Design review of the part shown in the three views and the two pictorial views. Dimensions are in mm from the part's minimum x, y and z. Give positions to 0.01 mm unless a question says otherwise; leave off trailing zeros. Loops run counter-clockwise (first coordinate to the right, second up) from the corner with the lowest first, then second, coordinate; pieces in that order, holes last. Notation, with made-up numbers: (-30, 42) -> (-4, 42) arc R5 ccw to (-4, 48) -> close; hole circle Ø8 at (21.5, 42). An arc over 180 degrees is marked (long way). One line per question, with ' | ' between items. Start each with the question number.
(1) Consider section A-A (z = 30.5). Write out the cut boundary in (x, y), and give its area (3 significant figures).
(2) Wall thickness on probe 1 along Y at (x, z) = (10, 77); probe 2 along X at (y, z) = (8.5, 61.5); probe 3 along Z at (x, y) = (10, 17.25): over which ranges is each line inside the solid? List them lowest first.
(3) Consider section B-B (z = 75). Write out the cut boundary in (x, y), and give its area (3 significant figures).
(4) Insertion check: P1, Ø1.5, axis at x = 15, y = 16, coming from the -Z side; P2, Ø1.5, axis at x = 17, z = 77, coming from the +Y side; P3, Ø6.5, axis at x = 10, y = 10, coming from the +Z side. Each pin has a flat end and moves straight along its axis. Give the tip position at first contact, or say it passes through.
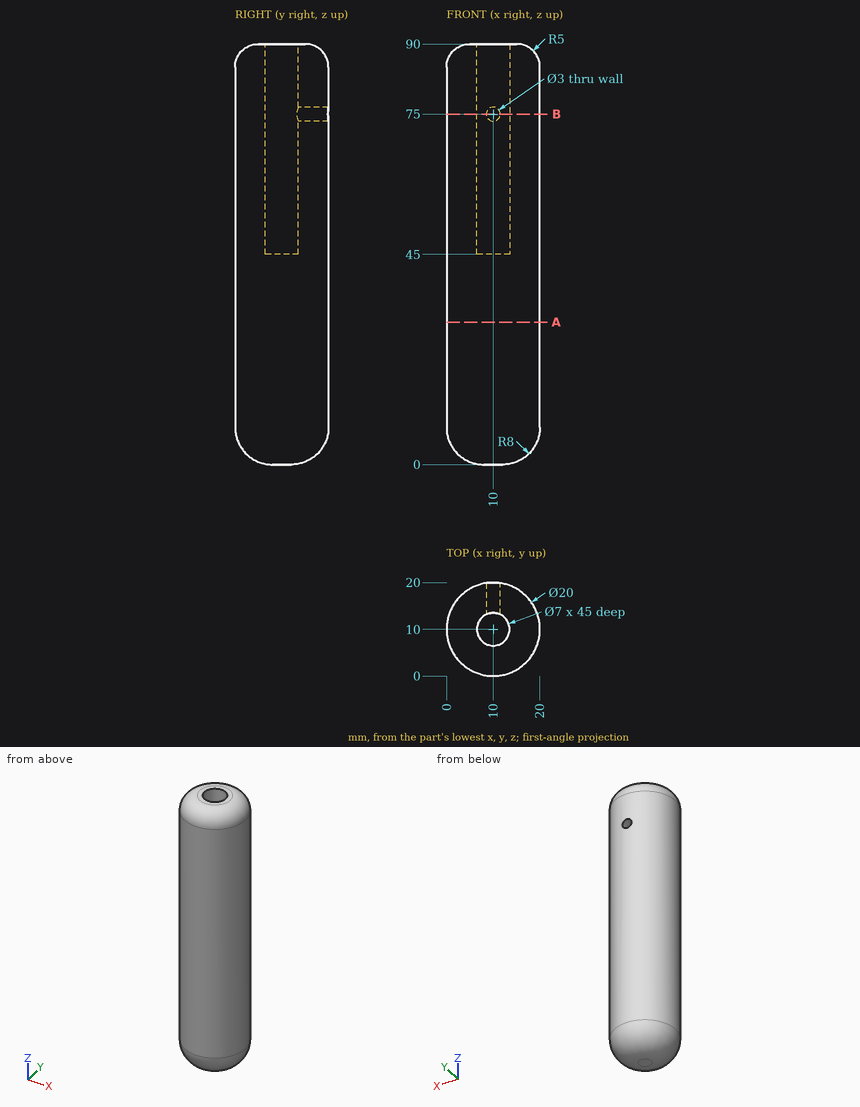
A:
1) outline: circle Ø20 at (10, 10) | area: 314 mm^2
2) probe 1: y = 0 to 6.5, 13.5 to 20 | probe 2: x = 0.11 to 6.84, 13.16 to 19.89 | probe 3: z = 1.96 to 73.5, 76.5 to 89.47
3) outline: (8.5, 13.16) -> (8.5, 19.89) arc R10 ccw (long way) to (11.5, 19.89) -> (11.5, 13.16) arc R3.5 cw (long way) to start | area: 256 mm^2
4) P1: stops at z = 1.8 | P2: stops at y = 17.81 | P3: stops at z = 45
